Source: three-view drawing plus pictorial views. Frame: mm from the lowest corner of the part. Give positions to 0.01 mm unless a question says otherwise; leave off trailing zeros. Order: outer loops, then holes, each group sorted by start corner. A loop starts at its lowest first (then second) coordinate and runs counter-clockwise, first axis right, second up.
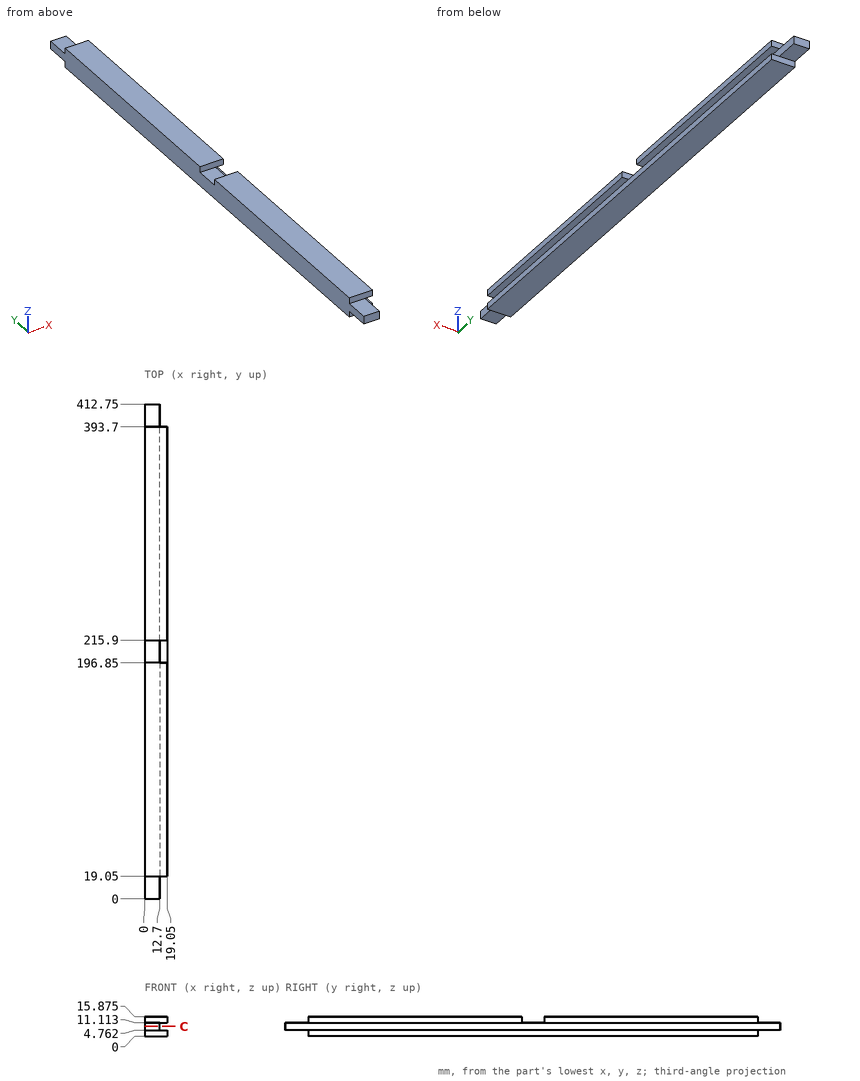
(1) Line query: line 1 along Y through (x, z) = (10.25, 14); line 2 along Z through (x, y) = (16.75, 164) (1 decimal); line 3 along X through (y, z) = (106, 5.5). Output: solid intervals per line, ascending.
(2) Section C-C, the plane z = 8. Return loops of the section in (x, y), plus the area to 3 significant figures.
(3) Pin query (flat end, axial travel): pin 1 Ø6.5 at (x, y) = (4.5, 13) entering from -Z; pin 2 Ø1.4 at (x, z) = (14, 2.5) entering from +Y; pin 3 Ø5 at (x, z) = (8, 13.5) entering from +Y; pin 4 Ø3 at (y, z) = (280, 8.5) entering from +X. Return the tip coordinate at first contact, or that it passes through.
Checks:
1. line 1: y = 19.05 to 196.85, 215.9 to 393.7
1. line 2: z = 0 to 4.8, 11.1 to 15.9
1. line 3: x = 0 to 12.7
2. outline: (0, 0) - (12.7, 0) - (12.7, 412.75) - (0, 412.75) - close
2. area: 5,240 mm2
3. pin 1: stops at z = 4.76
3. pin 2: stops at y = 393.7
3. pin 3: stops at y = 412.75
3. pin 4: stops at x = 12.7
